The model under review builds one solid part; all positions refer to its coordinate system, in mm. Coordinates: 2 decimals unless noted, no trailing zeros. Write each loop counter-clockwise with the first axis right and the second up, starting at its lowest first coordinate (ties: lowest second). Pieces come first, ordered by that corner, then holes. Notation, with made-up numbers: (67, -5.5) - (91, -5.5) arc R34 cw to (91, 32.5) - close; hole circle Ø9 at (0, -10.5). An arc over 180 degrees is marked (long way). Return JSON: item names as keys, results as strings. Group by question number.
(1) We need section B-B on z = 0.55. State the section outline as (x, y) points.
(2) We need section C-C on x = 0. State the section outline as (y, z) points, then the cut area to 3 significant figures.
(3) For pin 1 Ø2.5 at (x, y) = (23, -17.5) entering from +Z, flat-tipped, find the tip position at first contact; note if it passes through.
(4) We need section A-A on y = 20.5. State the section outline as (x, z) points, then the cut area to 3 significant figures.
(5) We need section D-D on y = -42.5. State the section outline as (x, z) points, then the cut area to 3 significant figures.
(6) To check wall thickness, follow L1, parallel to Y at x = 22.5, z = 1.05; L2, parallel to Y at x = -23, z = 2.2; L3, parallel to X at y = 25, z = 2.45. State the ranges of each line that lie inside material, in increasing order. Write a range as from..to.
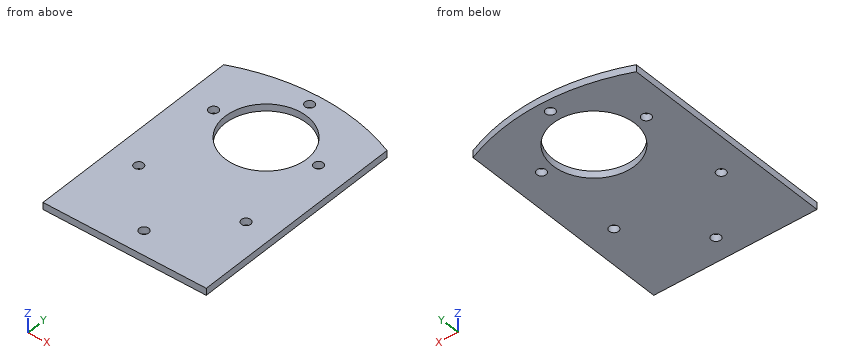
```python
from build123d import *

# Parameters (mm, degrees)
SKETCH1_W           = 70
SKETCH1_H           = 105
BOSS_EXTRUDE1_DEPTH = 3
SKETCH2_R           = 17.5
CUT_EXTRUDE3_DEPTH  = 3
SKETCH3_R           = 2
CUT_EXTRUDE4_DEPTH  = 3
SKETCH4_R           = 2
CUT_EXTRUDE5_DEPTH  = 5
CUT_EXTRUDE6_DEPTH  = 10


with BuildPart() as part:
    # Sketch1 → Boss-Extrude1 (new body)
    with BuildSketch(Plane.XY):
        Rectangle(SKETCH1_W, SKETCH1_H)
    extrude(amount=BOSS_EXTRUDE1_DEPTH)

    # Sketch2 → Cut-Extrude3 (cut)
    with BuildSketch(Plane(origin=(0, 0, 0), x_dir=(-1, 0, 0), z_dir=(0, 0, -1))):
        with Locations((0, 20.5)):
            Circle(SKETCH2_R)
    extrude(amount=-CUT_EXTRUDE3_DEPTH, mode=Mode.SUBTRACT)

    # Sketch3 → Cut-Extrude4 (cut)
    with BuildSketch(Plane.XY.offset(3)):
        with Locations((-22.5, 20.5)):
            Circle(SKETCH3_R)
        with Locations((0, 43)):
            Circle(SKETCH3_R)
        with Locations((22.5, 20.5)):
            Circle(SKETCH3_R)
    extrude(amount=-CUT_EXTRUDE4_DEPTH, mode=Mode.SUBTRACT)

    # Sketch4 → Cut-Extrude5 (cut)
    with BuildSketch(Plane.XY.offset(3)):
        with Locations((0, -42.5)):
            Circle(SKETCH4_R)
        with Locations((-23, -17.5)):
            Circle(SKETCH4_R)
        with Locations((23, -17.5)):
            Circle(SKETCH4_R)
    extrude(amount=-CUT_EXTRUDE5_DEPTH, mode=Mode.SUBTRACT)

    # Sketch5 → Cut-Extrude6 (cut)
    with BuildSketch(Plane.XY.offset(3)):
        with BuildLine():
            Line((-35, 40.793543502), (-35, 52.5))
            Line((-35, 52.5), (35, 52.5))
            Line((35, 52.5), (35, 40.793543502))
            ThreePointArc((35, 40.793543502), (0, 48.07644174), (-35, 40.793543502))
        make_face()
    extrude(amount=-CUT_EXTRUDE6_DEPTH, mode=Mode.SUBTRACT)


solid = part.part
```
Ans:
{
 "1": {"outline": "(-35, -52.5) - (35, -52.5) - (35, 40.79) arc R87.74 ccw to (-35, 40.79) - close; hole circle Ø4 at (-23, -17.5); hole circle Ø4 at (-22.5, 20.5); hole circle Ø35 at (0, 20.5); hole circle Ø4 at (0, -42.5); hole circle Ø4 at (0, 43); hole circle Ø4 at (22.5, 20.5); hole circle Ø4 at (23, -17.5)"},
 "2": {"outline": "(-52.5, 0) - (-44.5, 0) - (-44.5, 3) - (-52.5, 3) - close; (-40.5, 0) - (3, 0) - (3, 3) - (-40.5, 3) - close; (38, 0) - (41, 0) - (41, 3) - (38, 3) - close; (45, 0) - (48.08, 0) - (48.08, 3) - (45, 3) - close", "area": "173 mm²"},
 "3": {"pin 1": "through"},
 "4": {"outline": "(-35, 0) - (-24.5, 0) - (-24.5, 3) - (-35, 3) - close; (-20.5, 0) - (-17.5, 0) - (-17.5, 3) - (-20.5, 3) - close; (17.5, 0) - (20.5, 0) - (20.5, 3) - (17.5, 3) - close; (24.5, 0) - (35, 0) - (35, 3) - (24.5, 3) - close", "area": "81.0 mm²"},
 "5": {"outline": "(-35, 0) - (-2, 0) - (-2, 3) - (-35, 3) - close; (2, 0) - (35, 0) - (35, 3) - (2, 3) - close", "area": "198 mm²"},
 "6": {"L1": "-52.5..-19.44, -15.56..18.5, 22.5..45.14", "L2": "-52.5..-19.5, -15.5..18.56, 22.44..45.01", "L3": "-35..-16.91, 16.91..35"}
}
